The listing builds one solid part. Answer for the finished solid, in the listing's coordinates (mm). A direction names the side the tool comes from. Coordinates: 2 decimals unless noted, no trailing zeros. Order: outer loops, then holes, each group sorted by start corner. A loop starts at its lowest first (then second) coordinate and runs counter-clockwise, first axis right, second up.
Autodesk Inventor part; units mm, degrees
ref_plane "YZ Plane" through (0, 0, 0) normal (1, 0, 0) x (0, 1, 0)
ref_plane "XZ Plane" through (0, 0, 0) normal (0, 1, 0) x (-1, 0, 0)
ref_plane "XY Plane" through (0, 0, 0) normal (0, 0, 1) x (1, 0, 0)
sketch "스케치1" plane through (0, 0, 0) normal (0, 0, 1) x (1, 0, 0)
  circle A0 centre (0, 0) radius 46.25
  line L0 (-38.5, 38.5) -> (38.5, 38.5)
  line L1 (38.5, 38.5) -> (38.5, -38.5)
  line L2 (38.5, -38.5) -> (-38.5, -38.5)
  line L3 (-38.5, -38.5) -> (-38.5, 38.5)
  line L4 (-38.5, 38.5) -> (38.5, -38.5) construction
  line L5 (38.5, 38.5) -> (-38.5, -38.5) construction
  point P0 (-38.5, 25.6284)
  point P1 (-38.5, -25.6284)
  point P2 (-25.6284, -38.5)
  point P3 (25.6284, -38.5)
  point P4 (38.5, -25.6284)
  point P5 (38.5, 25.6284)
  point P6 (25.6284, 38.5)
  point P7 (-25.6284, 38.5)
  dimension "d0" = 92.5
  dimension "d1" = 77
  dimension "d2" = 77
extrude "돌출1" add sketch "스케치1" along normal blind 0.75 contours L1 A0 L2 L3 L0
sketch "스케치2" plane through (0, 0, 0) normal (0, 1, 0) x (-1, 0, 0)
  line L0 (25.6284, 0.75) -> (-25.6284, 0.75)
  line L1 (0, 0.75) -> (0, -28.2062)
  line L2 (38.5, 0) -> (38.5, -1.5)
  line L3 (38.5, -1.5) -> (35, -1.5)
  line L4 (35, -1.5) -> (35, -3.59)
  line L5 (35, -3.59) -> (0, -3.59)
  line L6 (38.5, 0) -> (25.6284, 0)
  line L7 (30, -3.59) -> (17.5, -9.59)
  line L8 (17.5, -9.59) -> (15, -11.99)
  line L9 (15, -11.99) -> (15, -21.99)
  line L10 (15, -21.99) -> (0, -21.99)
  line L11 (-25.6284, 0) -> (25.6284, 0)
  point P0 (0, 0)
  point P1 (0, 0)
  dimension "d5" = 1.5
  dimension "d6" = 2.09
  dimension "d7" = 77
  dimension "d8" = 70
  dimension "d9" = 60
  dimension "d10" = 35
  dimension "d11" = 30
  dimension "d12" = 6
  dimension "d13" = 2.4
  dimension "d14" = 10
revolve "회전1" add sketch "스케치2" angle 360 about axis through (0, 0, 0.75) along (0, 0, -1)
sketch "스케치3" plane through (0, 0, 0) normal (0, 1, 0) x (-1, 0, 0)
  line L0 (38.5, 0) -> (38.5, 0.75)
  line L1 (38.5, 0.75) -> (38.5, 1.75)
  line L2 (38.5, 1.75) -> (36.3, 1.75)
  line L3 (36.3, 1.75) -> (36.3, 0.75)
  line L4 (38.5, 0.75) -> (25.6284, 0.75)
  line L5 (9.1955, -2.25) -> (0, -2.25)
  line L6 (-35, -1.5) -> (35, -1.5)
  line L7 (0, -2.25) -> (0, 0.75)
  line L8 (25.6284, 0.75) -> (-25.6284, 0.75)
  line L9 (36.3, 0.75) -> (0, 0.75)
  line L10 (0, 0) -> (-25.6284, 0)
  line L11 (36.3, 0.75) -> (36.3, -0.45)
  line L12 (36.3, -0.45) -> (9.1955, -2.25)
  point P0 (20.489, -1.5)
  point P1 (0, -1.5)
  dimension "d16" = 1
  dimension "d17" = 2.2
  dimension "d18" = 1.2
  dimension "d19" = 3
revolve "회전2" add sketch "스케치3" angle 360 about axis through (0, 0, -2.25) along (0, 0, 1) contours L4 L3 L2 L1
revolve "회전3" cut sketch "스케치3" angle 360 about axis through (0, 0, -2.25) along (0, 0, 1) contours L11 L12 L6 L7 L8 L4 | L12 L5 L7 L6
sketch "스케치4" plane through (0, 0, 0.75) normal (0, 0, 1) x (1, 0, 0)
  circle A0 centre (0, 0) radius 42 construction
  line L0 (0, 0) -> (0, 16.8085)
  line L1 (0, 0) -> (-29.6985, 29.6985) construction
  line L2 (-29.6985, 29.6985) -> (-30.4056, 30.4056) construction
  line L3 (-28.2843, 31.1127) -> (-28.9914, 31.8198)
  line L4 (-31.8198, 28.9914) -> (-31.1127, 28.2843)
  arc A1 (-31.1127, 28.2843) -> (-28.2843, 31.1127) centre (-29.6985, 29.6985) ccw
  arc A2 (-28.9914, 31.8198) -> (-31.8198, 28.9914) centre (-30.4056, 30.4056) ccw
  point P0 (-30.052, 30.052)
  dimension "d22" = 84
  dimension "d23" = 45
  dimension "d24" = 1
  dimension "d25" = 4
extrude "돌출2" cut sketch "스케치4" against normal blind 0.75
pattern_circular "원형 패턴1" count 4 over 360 about axis through (0, 0, 1.25) along (0, 0, 1) of "돌출2"
properties part number "스피커"
1) Section A-A (z = -14.5) is taken. Give the vertices of the cut face in (x, y), then the cut area to 3 significant figures.
2) Consider L1, parallel to Y at x = 0, z = 0.2; L2, parallel to Y at x = -6.5, z = -7.75. Determine where each line is inside the solid, lowest interval first.
3) Determine the mould class of faces 1 (the face through (32.613, 32.794, 0.37)), 2 (the face through (28, -28, 0)), 3 (the face through (31.79, -31.85, 0.38)), 4 (the face through (0, 0, -2.25)) for opening direction X: released by +X, released by -X, zero draft, split by the parting line, or undercut.
4) Each of these flat-tipped pins is pushed along its axis until it touches: P1, Ø1.5, axis at x = 11.5, y = -3.5, coming from the +Z side; P2, Ø1.5, axis at x = -3.5, y = 1, coming from the +Z side; P3, Ø8, axis at x = -12, z = -13.5, coming from the +Y side. Where does it stop, or does it pass through?
5) Section B-B (z = -5.5) is taken. Give the vertices of the cut face in (x, y).
6) A tool of negligible diameter and unlimited length cuts with its end or side. For faces 5 (the face through (-29, 26, 0)), 6 (the face through (9, -34, -1.5)), 7 (the face through (28, -28, 0.75)), 8 (the face through (-29, -26, 0.75)), from which of +Z, -Z, +X, -X, +Y, -Y can it reach the whole face along a straight path? Write none if from no direction.
Filled sheet:
1. outline: circle Ø30 at (0, 0)
1. area: 707 mm2
2. L1: y = -38.5 to -36.3, 36.3 to 38.5
2. L2: y = -20.32 to 20.32
3. face 1: released by +X
3. face 2: zero draft
3. face 3: undercut
3. face 4: undercut
4. P1: stops at z = -2.01
4. P2: stops at z = -2.25
4. P3: stops at y = 13.79
5. outline: circle Ø52.04 at (0, 0)
6. face 5: -Z, -X, +Y
6. face 6: -Z
6. face 7: +Z, +X, -Y
6. face 8: +Z, -X, -Y
